Geometry check sheet. Reference: drawing and pictorial views, mm from the part's lowest x, y, z. A direction names the side the tool comes from. Coordinates: 2 decimals unless noted, no trailing zeros. Loops run counter-clockwise (first coordinate to the right, second up) from the corner with the lowest first, then second, coordinate; pieces in that order, holes last.
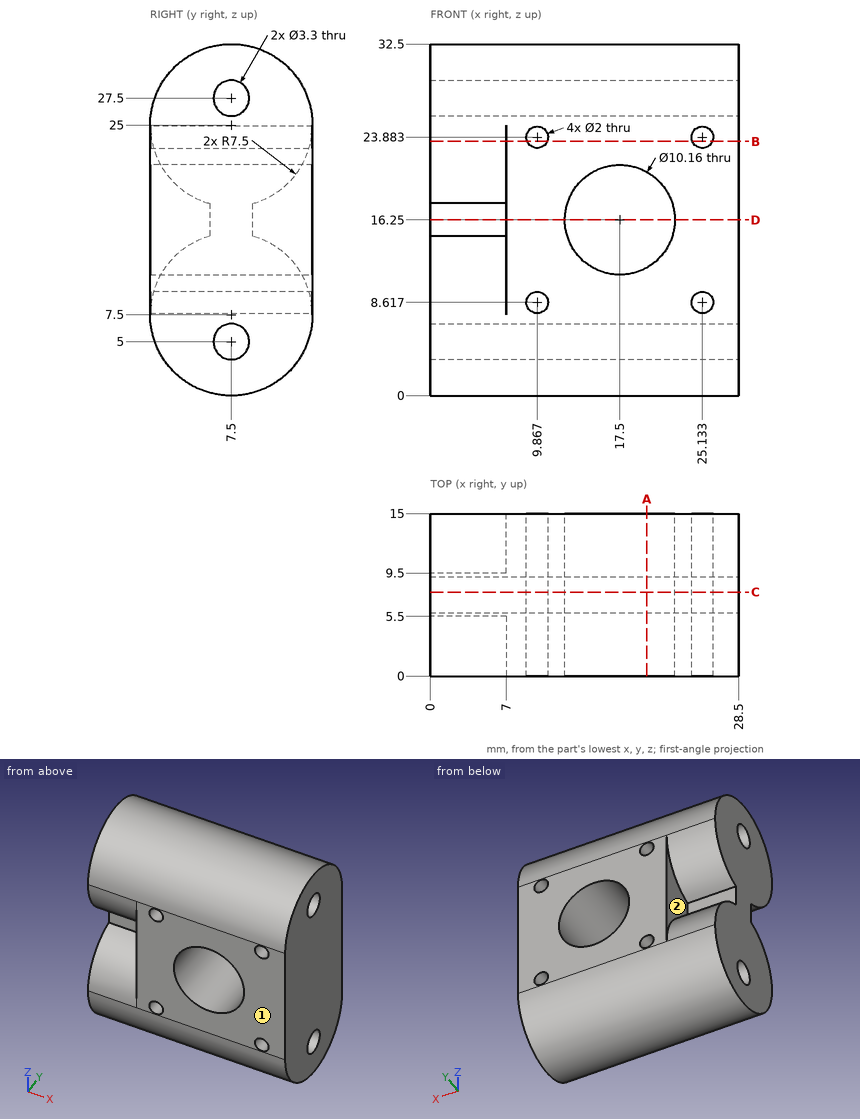
1) Access from +Z, -Z, +X, -X, +Y, -Y to the whole of each face (thin tool, end or side, straight path). Record for the marked faces 1 and 2.
Data:
face 1: +Z, -Z, +X, -X, -Y
face 2: -X, +Y
2) Section check D-D on z = 16.25. Record the cut outline in (x, y), and give its area (3 significant figures).
Data:
outline: (0, 5.5) - (7, 5.5) - (7, 0) - (12.42, 0) - (12.42, 15) - (7, 15) - (7, 9.5) - (0, 9.5) - close; (22.58, 0) - (28.5, 0) - (28.5, 15) - (22.58, 15) - close
area: 198 mm2
3) Depth check by flat-ended pin: pin 1 (1.5 mm diameter, centred on x = 2.5, z = 16, fed in from -Y); pin 2 (1.5 mm diameter, centred on y = 3, z = 21, fed in from -X); pin 3 (6 mm diameter, centred on x = 17.5, z = 16.25, fed in from +Y); pin 4 (3 mm diameter, centred on x = 23.5, z = 27, fed in from +Y). Enter the tip coordinate at first touch or a pass-through.
Data:
pin 1: stops at y = 5.5
pin 2: stops at x = 0
pin 3: passes through
pin 4: stops at y = 14.98
4) Material ranges on probe 1 along Z at (x, y) = (24.5, 13.25); probe 2 along Z at (x, y) = (15.75, 7.5); probe 3 along Z at (x, y) = (9.25, 14), recorded low to high.
Data:
probe 1: z = 2.68 to 7.84, 9.39 to 23.11, 24.66 to 29.82
probe 2: z = 0 to 3.35, 6.65 to 11.48, 21.02 to 25.85, 29.15 to 32.5
probe 3: z = 3.76 to 7.83, 9.4 to 23.1, 24.67 to 28.74
5) Section check C-C on y = 7.75. Record the cut outline in (x, z), and give its area (3 significant figures).
Data:
outline: (0, 0) - (28.5, 0) - (28.5, 3.37) - (0, 3.37) - close; (0, 6.63) - (28.5, 6.63) - (28.5, 25.87) - (0, 25.87) - close; (0, 29.13) - (28.5, 29.13) - (28.5, 32.5) - (0, 32.5) - close; hole circle Ø2 at (9.87, 8.62); hole circle Ø2 at (9.87, 23.88); hole circle Ø10.16 at (17.5, 16.25); hole circle Ø2 at (25.13, 8.62); hole circle Ø2 at (25.13, 23.88)
area: 646 mm2
6) Section check B-B on z = 23.5. Record the cut outline in (x, y), and give its area (3 significant figures).
Data:
outline: (0, 0.15) - (7, 0.15) - (7, 0) - (8.94, 0) - (8.94, 15) - (7, 15) - (7, 14.85) - (0, 14.85) - close; (10.79, 0) - (24.21, 0) - (24.21, 15) - (10.79, 15) - close; (26.06, 0) - (28.5, 0) - (28.5, 15) - (26.06, 15) - close
area: 370 mm2
7) Section check A-A on x = 20. Record the cut outline in (y, z).
Data:
outline: (0, 7.5) arc R7.5 ccw to (15, 7.5) - (15, 11.83) - (0, 11.83) - close; (0, 20.67) - (15, 20.67) - (15, 25) arc R7.5 ccw to (0, 25) - close; hole circle Ø3.3 at (7.5, 5); hole circle Ø3.3 at (7.5, 27.5)
